Geometry: final body of the model. Coordinates: model frame, mm. A direction names the side the tool comes from. Give positions to 0.01 mm unless a question says otherwise; leave off trailing zeros. Write each loop counter-clockwise with the first axis right and the second up, starting at its lowest first coordinate (ties: lowest second). Pieces come first, ordered by that corner, then holes.
```python
from build123d import *

# Parameters (mm, degrees)
BOSS_EXTRUDE1_DEPTH = 3
FILLET1_R           = 0.5


with BuildPart() as part:
    # Sketch1 → Boss-Extrude1 (new body)
    with BuildSketch(Plane(origin=(0, 0, 0), x_dir=(1, 0, 0), z_dir=(0, 1, 0))):
        with BuildLine():
            Line((-12, 7), (12, 7))
            ThreePointArc((12, 7), (14.828427125, 5.828427125), (16, 3))
            Line((16, 3), (16, -3))
            ThreePointArc((16, -3), (14.828427125, -5.828427125), (12, -7))
            Line((12, -7), (-12, -7))
            ThreePointArc((-12, -7), (-14.828427125, -5.828427125), (-16, -3))
            Line((-16, -3), (-16, 3))
            ThreePointArc((-16, 3), (-14.828427125, 5.828427125), (-12, 7))
        make_face()
        with BuildLine():
            Line((-12, 4), (12, 4))
            ThreePointArc((12, 4), (12.707106781, 3.707106781), (13, 3))
            Line((13, 3), (13, -3))
            ThreePointArc((13, -3), (12.707106781, -3.707106781), (12, -4))
            Line((12, -4), (-12, -4))
            ThreePointArc((-12, -4), (-12.707106781, -3.707106781), (-13, -3))
            Line((-13, -3), (-13, 3))
            ThreePointArc((-13, 3), (-12.707106781, 3.707106781), (-12, 4))
        make_face(mode=Mode.SUBTRACT)
    extrude(amount=BOSS_EXTRUDE1_DEPTH)

    # Fillet1
    fillet1_edges = [part.edges().sort_by_distance(p)[0] for p in [
        (-14.828427125, 3, 5.828427125),
        (-16, 0, 0),
        (-14.828427125, 0, -5.828427125),
        (0, 3, 7),
        (14.828427125, 3, 5.828427125),
        (16, 3, 0),
        (14.828427125, 3, -5.828427125),
        (0, 3, -7),
        (12.707106781, 0, -3.707106781),
        (0, 0, -4),
        (-12.707106781, 0, -3.707106781),
        (-13, 0, 0),
        (-12.707106781, 0, 3.707106781),
        (0, 0, 4),
        (12.707106781, 0, 3.707106781),
        (13, 0, 0),
        (12.707106781, 3, -3.707106781),
        (0, 3, -4),
        (-12.707106781, 3, -3.707106781),
        (-13, 3, 0),
        (-12.707106781, 3, 3.707106781),
        (0, 3, 4),
        (12.707106781, 3, 3.707106781),
        (13, 3, 0),
        (-14.828427125, 3, -5.828427125),
        (-16, 3, 0),
        (0, 0, -7),
        (14.828427125, 0, -5.828427125),
        (16, 0, 0),
        (14.828427125, 0, 5.828427125),
        (0, 0, 7),
        (-14.828427125, 0, 5.828427125),
    ]]
    fillet(fillet1_edges, radius=FILLET1_R)


solid = part.part
```
Item 1: Pull-direction query (X, two-part tool) for faces 1 (the face through (14.859, 1.486, 5.797)), 2 (the face through (0, 1, 4)), 3 (the face through (0, 1, 7)); classes: +X half, -X half, draft (parallel to the pull), parting line (faces both ways), or undercut.
Found:
face 1: +X half
face 2: undercut
face 3: draft
Item 2: Section A-A, the plane z = 0.5. Return the cut outline in (x, y).
Found:
outline: (-16, 0.5) arc R0.5 ccw to (-15.5, 0) - (-13.5, 0) arc R0.5 ccw to (-13, 0.5) - (-13, 2.5) arc R0.5 ccw to (-13.5, 3) - (-15.5, 3) arc R0.5 ccw to (-16, 2.5) - close; (13, 0.5) arc R0.5 ccw to (13.5, 0) - (15.5, 0) arc R0.5 ccw to (16, 0.5) - (16, 2.5) arc R0.5 ccw to (15.5, 3) - (13.5, 3) arc R0.5 ccw to (13, 2.5) - close
Item 3: Section C-C, the plane y = 0.8. Return the cut outline in (x, z).
Found:
outline: (-16, -3) arc R4 ccw to (-12, -7) - (12, -7) arc R4 ccw to (16, -3) - (16, 3) arc R4 ccw to (12, 7) - (-12, 7) arc R4 ccw to (-16, 3) - close; hole (-13, -3) arc R1 ccw to (-12, -4) - (12, -4) arc R1 ccw to (13, -3) - (13, 3) arc R1 ccw to (12, 4) - (-12, 4) arc R1 ccw to (-13, 3) - close
Item 4: Pin query (flat end, axial travel): pin 1 Ø6 at (x, z) = (-7.5, 0) entering from +Y. Return the tip coordinate at first contact, or that it passes through.
Found:
pin 1: passes through
Item 5: Line query: L1, parallel to Z at x = -7, y = 0.8; L2, parallel to X at y = 1.9, z = 0.5; L3, parallel to X at y = 0.1, z = 2. Output: solid intervals per line, ascending.
Found:
L1: z = -7 to -4, 4 to 7
L2: x = -16 to -13, 13 to 16
L3: x = -15.8 to -13.2, 13.2 to 15.8
Item 6: Reachability of faces 4 (the face through (-14.859, 1.486, -5.797)), 5 (the face through (12.715, 1.486, 3.699)) from +Z, -Z, +X, -X, +Y, -Y: full face, straight path, thin tool, end or side. Return the list, or none.
Found:
face 4: -Z, -X, +Y, -Y
face 5: +Y, -Y
Item 7: Section B-B, the plane x = -8. Return the cut outline in (y, z).
Found:
outline: (0, -6.5) arc R0.5 ccw to (0.5, -7) - (2.5, -7) arc R0.5 ccw to (3, -6.5) - (3, -4.5) arc R0.5 ccw to (2.5, -4) - (0.5, -4) arc R0.5 ccw to (0, -4.5) - close; (0, 4.5) arc R0.5 ccw to (0.5, 4) - (2.5, 4) arc R0.5 ccw to (3, 4.5) - (3, 6.5) arc R0.5 ccw to (2.5, 7) - (0.5, 7) arc R0.5 ccw to (0, 6.5) - close
